Source: CAD feature listing. Evaluate the final solid. Frame: model axes, mm. A direction names the side the tool comes from. Give positions to 0.01 mm unless a question says otherwise; leave off trailing zeros. Write each loop counter-clockwise with the first axis right and the second up, starting at its lowest first coordinate (ties: lowest second). Pieces come first, ordered by that corner, then holes. Notation, with made-up numbers: M 78,77 L 87,77 A17 ccw 87,99 Z; hole C 20.25,11.5 d7. An arc over 180 degrees is marked long. Return JSON: item names as keys, results as strings.
```python
from build123d import *

# Parameters (mm, degrees)
BOSS_EXTRUDE1_DEPTH = 4
CUT_EXTRUDE1_DEPTH  = 2
BOSS_EXTRUDE2_DEPTH = 10
SKETCH4_R           = 3
BOSS_EXTRUDE3_DEPTH = 4
SKETCH5_R           = 2.5
CUT_EXTRUDE2_DEPTH  = 3
CHAMFER1_SIZE       = 1
SKETCH6_W           = 2
SKETCH6_H           = 4
BOSS_EXTRUDE4_DEPTH = 5
FILLET1_R           = 10
CUT_EXTRUDE3_DEPTH  = 10


with BuildPart() as part:
    # Sketch1 → Boss-Extrude1 (new body)
    with BuildSketch(Plane(origin=(0, 0, 0), x_dir=(1, 0, 0), z_dir=(0, 1, 0))):
        with BuildLine():
            Line((-8.269520907, -3.551763501), (-5.5, -10))
            Line((-5.5, -10), (5.5, -10))
            Line((5.5, -10), (8.269520907, -3.551763501))
            ThreePointArc((8.269520907, -3.551763501), (0, 9), (-8.269520907, -3.551763501))
        make_face()
    extrude(amount=BOSS_EXTRUDE1_DEPTH)

    # Sketch2 → Cut-Extrude1 (cut)
    with BuildSketch(Plane(origin=(0, 4, 0), x_dir=(1, 0, 0), z_dir=(0, 1, 0))):
        with BuildLine():
            Line((-6.753885149, -3.261140198), (-3.5, -10))
            Line((-3.5, -10), (3.5, -10))
            Line((3.5, -10), (6.753885149, -3.261140198))
            ThreePointArc((6.753885149, -3.261140198), (0, 7.5), (-6.753885149, -3.261140198))
        make_face()
    extrude(amount=-CUT_EXTRUDE1_DEPTH, mode=Mode.SUBTRACT)

    # Sketch3 → Boss-Extrude2 (add)
    with BuildSketch(Plane.XZ):
        with BuildLine():
            Line((-1.717556404, 0.975), (1.717556404, 0.975))
            ThreePointArc((1.717556404, 0.975), (0, -1.975), (-1.717556404, 0.975))
        make_face()
    extrude(amount=BOSS_EXTRUDE2_DEPTH)

    # Sketch4 → Boss-Extrude3 (add)
    with BuildSketch(Plane.XZ):
        with Locations(Location((0, 0, 0), (0, 0, 90))):
            Circle(SKETCH4_R)
    extrude(amount=BOSS_EXTRUDE3_DEPTH)

    # Sketch5 → Cut-Extrude2 (cut)
    with BuildSketch(Plane(origin=(0, 2, 0), x_dir=(1, 0, 0), z_dir=(0, 1, 0))):
        with Locations(Location((0, 0, 0), (0, 0, 270))):
            Circle(SKETCH5_R)
    extrude(amount=-CUT_EXTRUDE2_DEPTH, mode=Mode.SUBTRACT)

    # Chamfer1
    chamfer1_edges = [part.edges().sort_by_distance(p)[0] for p in [
        (0, 0, -3),
        (0, -4, -3),
    ]]
    chamfer(chamfer1_edges, length=CHAMFER1_SIZE)

    # Sketch6 → Boss-Extrude4 (add)
    with BuildSketch(Plane.XY.offset(10)):
        with Locations((4.5, 2)):
            Rectangle(SKETCH6_W, SKETCH6_H)
    extrude(amount=BOSS_EXTRUDE4_DEPTH)

    # Fillet1
    fillet1_edges = [part.edges().sort_by_distance(p)[0] for p in [
        (3.5, 3, 10),
    ]]
    fillet(fillet1_edges, radius=FILLET1_R)

    # Sketch8 → Cut-Extrude3 (cut)
    with BuildSketch(Plane.XZ):
        Polygon((-5.5, 10), (-1.5, 10), (-8.511399863, 2.988600137), align=None)
    extrude(amount=-CUT_EXTRUDE3_DEPTH, mode=Mode.SUBTRACT)


solid = part.part
```
1) Cut plane A-A, the plane y = 0.5. Return the cut outline in (x, z).
Numbers:
{"outline": "M -8.48,3.02 A9 ccw long 8.27,3.55 L 5.5,10 L 5.5,15 L 3.5,15 L 3.5,10 L -1.5,10 Z; hole C 0,0 d5"}
2) Cut plane C-C, the plane x = 0. Return the cut outline in (y, z) (3 decimals), then the cut area to 3 significant figures.
Numbers:
{"outline": "M -10,-1.975 L -4,-1.975 L -4,-2 L -3,-3 L -1,-3 L 0,-4 L 0,-9 L 4,-9 L 4,-7.5 L 2,-7.5 L 2,-2.5 L -1,-2.5 L -1,2.5 L 2,2.5 L 2,10 L 0,10 L 0,4 L -1,3 L -3,3 L -4,2 L -4,0.975 L -10,0.975 Z", "area": "67.7 mm²"}
3) Set-up query: faces 4 (the face through (0, -7, 0.975)), 5 (the face through (5.5, 2, 12)), 6 (the face through (2, 2, 2)), 7 (the face through (4, 0, 3)), 8 (the face through (3.745, 2.986, 10.088)). Return all of +Z, -Z, +X, -X, +Y, -Y with unobstructed straight access to the full face (end or side cutting, diameter ignored); none if empty.
Numbers:
{"face 4": "+Z, +X, -X, -Y", "face 5": "+Z, +X, +Y, -Y", "face 6": "+Y", "face 7": "-Y", "face 8": "-X, +Y"}
4) Contact query for flat-ended pins moving along their axis: pin 1 Ø6 at (y, z) = (2, 8) entering from -X; pin 2 Ø1.7 at (x, y) = (0.5, -7.5) entering from +Z (3 decimals); pin 3 Ø5 at (x, y) = (0, -4) entering from +Z. Output: stop coordinate, or through.
Numbers:
{"pin 1": "stops at x = -6.5", "pin 2": "stops at z = 0.975", "pin 3": "stops at z = 3"}
5) Cut plane D-D, the plane y = -3.5. Return the cut outline in (x, z), then the cut area to 3 significant figures.
Numbers:
{"outline": "C 0,0 d5", "area": "19.6 mm²"}
6) Cut plane B-B, the plane z = 0. Return the cut outline in (x, y) (3 decimals), then the cut area to 3 significant figures.
Numbers:
{"outline": "M -9,0 L -4,0 L -3,-1 L -3,-3 L -2,-4 L -1.975,-4 L -1.975,-10 L 1.975,-10 L 1.975,-4 L 2,-4 L 3,-3 L 3,-1 L 4,0 L 9,0 L 9,4 L 7.5,4 L 7.5,2 L 2.5,2 L 2.5,-1 L -2.5,-1 L -2.5,2 L -7.5,2 L -7.5,4 L -9,4 Z", "area": "74.7 mm²"}
7) Draft query along X for faces 1 (the face through (1, 1, 10)), 2 (the face through (5.61, 3.01, 5.63)), 3 (the face through (3.5, 2, 13)). Return one class per face: released by +X, released by -X, zero draft, split by the parting line, or undercut.
Numbers:
{"face 1": "zero draft", "face 2": "undercut", "face 3": "released by -X"}
8) Line query: line 1 (X direction, y = 0.45, z = 0); line 2 (Y direction, x = -3.75, z = -2); line 3 (Y direction, x = 1, z = -7.5). Output: solid intervals per line, ascending. Write a range as [from, to].
Numbers:
{"line 1": "x = [-9, -2.5], [2.5, 9]", "line 2": "y = [0, 2]", "line 3": "y = [0, 4]"}
